Study the drawing (mm; zero at the part's minimum x, y, z) and answer. Give positions to 0.01 mm unless a question says otherwise; leave off trailing zeros. Write each loop counter-clockwise with the first axis right and the second up, starting at its lowest first coordinate (ties: lowest second). Pieces come first, ordered by that corner, then holes. Notation, with made-up numbers: (-24, 63.5) - (-8, 63.5) arc R22 cw to (-8, 78.5) - close; hole circle Ø7 at (4, 76.25). An arc over 180 degrees is marked (long way). One line per item, written item: value. Start each with the question number.
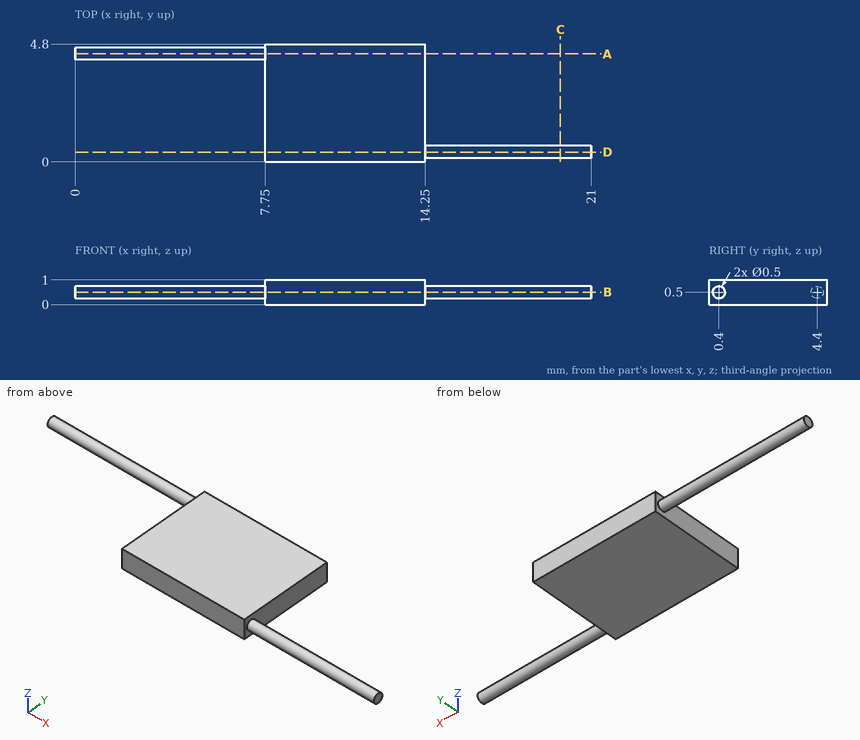
Item 1: Find section B-B on z = 0.5. Determine the outline of the cut face in (x, y).
Item 2: Find section C-C on x = 19.75. Determine the outline of the cut face in (y, z).
Item 3: Find section A-A on y = 4.4. Determine the outline of the cut face in (x, z), plus the area to 3 significant figures.
Item 4: Find section D-D on y = 0.4. Determine the outline of the cut face in (x, z).
Item 5: Straight lines are drawn through the part: line 1 along X through (y, z) = (3.9, 0.1); line 2 along X through (y, z) = (4.4, 0.3); line 3 along Y through (x, z) = (16, 0.55). For each, find the intervals that lie inside material, in ascending order.
Values:
1. outline: (0, 4.15) - (7.75, 4.15) - (7.75, 0) - (14.25, 0) - (14.25, 0.15) - (21, 0.15) - (21, 0.65) - (14.25, 0.65) - (14.25, 4.8) - (7.75, 4.8) - (7.75, 4.65) - (0, 4.65) - close
2. outline: circle Ø0.5 at (0.4, 0.5)
3. outline: (0, 0.25) - (7.75, 0.25) - (7.75, 0) - (14.25, 0) - (14.25, 1) - (7.75, 1) - (7.75, 0.75) - (0, 0.75) - close
3. area: 10.4 mm^2
4. outline: (7.75, 0) - (14.25, 0) - (14.25, 0.25) - (21, 0.25) - (21, 0.75) - (14.25, 0.75) - (14.25, 1) - (7.75, 1) - close
5. line 1: 7.75 to 14.25
5. line 2: 0 to 14.25
5. line 3: 0.16 to 0.64
